```python
from build123d import *

# Parameters (mm, degrees)
ESQUISSE1_W             = 20
ESQUISSE1_H             = 3
BOSS_EXTRU_1_DEPTH      = 3
ESQUISSE2_W             = 172
ESQUISSE2_H             = 1
ENL_V_MAT_EXTRU_1_DEPTH = 1.5
ESQUISSE4_W             = 3
ESQUISSE4_H             = 20
ENL_V_MAT_EXTRU_2_DEPTH = 207.455986147
ESQUISSE5_W             = 70
ESQUISSE5_H             = 100
BOSS_EXTRU_2_DEPTH      = 25
ESQUISSE6_W             = 62
ESQUISSE6_H             = 22.5
ENL_V_MAT_EXTRU_3_DEPTH = 95
ESQUISSE10_W            = 30
ESQUISSE10_H            = 50
BOSS_EXTRU_3_DEPTH      = 20
ESQUISSE11_W            = 25
ESQUISSE11_H            = 17.5
ENL_V_MAT_EXTRU_5_DEPTH = 47
ESQUISSE12_W            = 8
ESQUISSE12_H            = 22.5
BOSS_EXTRU_5_DEPTH      = 15
ESQUISSE15_W            = 7.5
ESQUISSE15_H            = 20
ENL_V_MAT_EXTRU_7_DEPTH = 15
ENL_V_MAT_EXTRU_8_REACH = 210.324
ESQUISSE17_W            = 9
ESQUISSE17_H            = 15
ENL_V_MAT_EXTRU_9_DEPTH = 10


with BuildPart() as part:
    # Esquisse1 → Boss.-Extru.1 (new body)
    with BuildSketch(Plane.XY):
        with BuildLine():
            Line((-109.499197329, 0), (62.500802671, 0))
            Line((62.500802671, 0), (62.500802671, -175))
            Line((62.500802671, -175), (56.500802671, -175))
            ThreePointArc((56.500802671, -175), (-23.499197329, -130.484780132), (-103.499197329, -175))
            Line((-103.499197329, -175), (-109.499197329, -175))
            Line((-109.499197329, -175), (-109.499197329, 0))
        make_face()
        with Locations((-83.499197329, -123.5)):
            Rectangle(ESQUISSE1_W, ESQUISSE1_H, mode=Mode.SUBTRACT)
        with Locations((-23.499197329, -123.5)):
            Rectangle(ESQUISSE1_W, ESQUISSE1_H, mode=Mode.SUBTRACT)
        with Locations((36.500802671, -123.5)):
            Rectangle(ESQUISSE1_W, ESQUISSE1_H, mode=Mode.SUBTRACT)
    extrude(amount=BOSS_EXTRU_1_DEPTH)

    # Esquisse2 → Enlèv. mat.-Extru.1 (cut)
    with BuildSketch(Plane.XY.offset(3)):
        with Locations((-23.499197329, -1)):
            Rectangle(ESQUISSE2_W, ESQUISSE2_H)
    extrude(amount=-ENL_V_MAT_EXTRU_1_DEPTH, mode=Mode.SUBTRACT)

    # Esquisse4 → Enlèv. mat.-Extru.2 (cut, through all)
    with BuildSketch(Plane.XY.offset(3)):
        with Locations((-107.999197329, -78.25)):
            Rectangle(ESQUISSE4_W, ESQUISSE4_H)
        with Locations((61.000802671, -78.25)):
            Rectangle(ESQUISSE4_W, ESQUISSE4_H)
    extrude(amount=-ENL_V_MAT_EXTRU_2_DEPTH, mode=Mode.SUBTRACT)

    # Esquisse5 → Boss.-Extru.2 (add)
    with BuildSketch(Plane.XY.offset(3)):
        with Locations((-22.499197329, -66.5)):
            Rectangle(ESQUISSE5_W, ESQUISSE5_H)
    extrude(amount=BOSS_EXTRU_2_DEPTH)

    # Esquisse6 → Enlèv. mat.-Extru.3 (cut)
    with BuildSketch(Plane(origin=(0, -16.5, 0), x_dir=(1, 0, 0), z_dir=(0, 1, 0))):
        with Locations((-22.499197329, -14.25)):
            Rectangle(ESQUISSE6_W, ESQUISSE6_H)
    extrude(amount=-ENL_V_MAT_EXTRU_3_DEPTH, mode=Mode.SUBTRACT)

    # Esquisse10 → Boss.-Extru.3 (add)
    with BuildSketch(Plane.XY.offset(3)):
        with Locations((-72.499197329, -91.5)):
            Rectangle(ESQUISSE10_W, ESQUISSE10_H)
    extrude(amount=BOSS_EXTRU_3_DEPTH)

    # Esquisse11 → Enlèv. mat.-Extru.5 (cut)
    with BuildSketch(Plane(origin=(0, -66.5, 0), x_dir=(1, 0, 0), z_dir=(0, 1, 0))):
        with Locations((-72.499197329, -11.75)):
            Rectangle(ESQUISSE11_W, ESQUISSE11_H)
    extrude(amount=-ENL_V_MAT_EXTRU_5_DEPTH, mode=Mode.SUBTRACT)

    # Esquisse12 → Boss.-Extru.5 (add)
    with BuildSketch(Plane(origin=(12.500802671, 0, 0), x_dir=(0, 0, -1), z_dir=(1, 0, 0))):
        with Locations((-7, -100.25)):
            Rectangle(ESQUISSE12_W, ESQUISSE12_H)
    extrude(amount=BOSS_EXTRU_5_DEPTH)

    # Esquisse15 → Enlèv. mat.-Extru.7 (cut)
    with BuildSketch(Plane.ZY.offset(-8.500802671)):
        with Locations((6.75, -100.25)):
            Rectangle(ESQUISSE15_W, ESQUISSE15_H)
    extrude(amount=-ENL_V_MAT_EXTRU_7_DEPTH, mode=Mode.SUBTRACT)

    # Esquisse17 → Enlèv. mat.-Extru.8 (cut, up to next)
    with BuildSketch(Plane(origin=(0, 0, 0), x_dir=(-1, 0, 0), z_dir=(0, 0, -1)), mode=Mode.PRIVATE) as enl_v_mat_extru_8_sk1:
        with Locations((-19.000802671, -99.5)):
            Rectangle(ESQUISSE17_W, ESQUISSE17_H)
    enl_v_mat_extru_8_tool1 = extrude(enl_v_mat_extru_8_sk1.sketch, amount=-ENL_V_MAT_EXTRU_8_REACH, mode=Mode.PRIVATE) & part.part
    add(enl_v_mat_extru_8_tool1.solids().sort_by_distance((19.000803, -99.5, 0))[0], mode=Mode.SUBTRACT)

    # Esquisse18 → Enlèv. mat.-Extru.9 (cut)
    with BuildSketch(Plane.XY.offset(3)):
        with BuildLine():
            ThreePointArc((-8.555469882, -131.678386461), (-22.519051553, -117.45703568), (-36.740402335, -131.420617351))
            Line((-36.740402335, -131.420617351), (-8.555469882, -131.678386461))
        make_face()
    extrude(amount=-ENL_V_MAT_EXTRU_9_DEPTH, mode=Mode.SUBTRACT)


solid = part.part
```
Geometry check sheet. Reference: the model listing, model coordinates, mm. A direction names the side the tool comes from. Round coordinates to 2 decimals unless told otherwise and drop trailing zeros. Order: outer loops, then holes, each group sorted by start corner. A loop starts at its lowest first (then second) coordinate and runs counter-clockwise, first axis right, second up. Notation, with made-up numbers: (-35.5, 23.25) - (-2.5, 23.25) arc R24 cw to (-2.5, 58.25) - close; hole circle Ø5 at (51, -17). An arc over 180 degrees is marked (long way). Use a Markdown table: item, result. Add a question column.
1) Thickness scan on line 1 along Z through (x, y) = (-46, -59); line 2 along X through (y, z) = (-111, 6); line 3 along Z through (x, y) = (-61, -97.5). Record the ranges inside material, lowest first.
2) Set-up check for faces 1 (the flat face through (-73, -90, 20.5)), 2 (the cylindrical face through (29.15, -146.583, 1.479)), 3 (the flat face through (-28, -16.5, 26)), 4 (the flat face through (20, -89, 7)), 5 (the flat face through (-87.499, -92, 13)): record each of +Z, -Z, +X, -X, +Y, -Y from which the full face is reachable in a straight line by a thin tool's end or side.
3) Section check B-B (x = 44.5). Record the cut outline in (y, z), then the cut area to 3 significant figures.
4) Mould release check, pull along Y, two halves, no side actions. Record for faces 6 (the flat face through (-23, -111.5, 14)), 7 (the cylindrical face through (-74.477, -145.481, 1.479)), 8 (the flat face through (-23, -63, 25.5)), 9 (the flat face through (16, -110.25, 7)): released by +Y, released by -Y, zero draft, split by the parting line, or undercut.
5) Section check C-C (y = -157). Record the cut outline in (x, z).
6) Section check D-D (x = 19). Record the cut outline in (y, z), then the cut area to 3 significant figures.
7) Gauge pin test, flat ends, axial feed: P1, Ø7.5, axis at y = -87.5, z = 12, coming from the -X side; P2, Ø8, axis at y = -67.5, z = 18.5, coming from the +X side; P3, Ø6, axis at x = -9.5, z = 15, coming from the +Y side. Record the tip position at first contact, or that the pin passes through.
8) Section check A-A (y = -72). Record the cut outline in (x, z), then the cut area to 3 significant figures.
Established:
| question | item | result |
|---|---|---|
| 1 | line 1 | 0 to 3, 25.5 to 28 |
| 1 | line 2 | -87.5 to -85, -60 to -53.5, 8.5 to 27.5 |
| 1 | line 3 | 0 to 3, 20.5 to 23 |
| 2 | face 1 | +Y |
| 2 | face 2 | +Z, -Z, -Y |
| 2 | face 3 | +Z, +X, -X, +Y |
| 2 | face 4 | +Z, +X, +Y |
| 2 | face 5 | +Z, -X, +Y, -Y |
| 3 | outline | (-159.52, 0) - (-125, 0) - (-125, 3) - (-159.52, 3) - close; (-122, 0) - (0, 0) - (0, 3) - (-0.5, 3) - (-0.5, 1.5) - (-1.5, 1.5) - (-1.5, 3) - (-122, 3) - close |
| 3 | area | 468 mm2 |
| 4 | face 6 | released by +Y |
| 4 | face 7 | released by -Y |
| 4 | face 8 | zero draft |
| 4 | face 9 | undercut |
| 5 | outline | (-109.5, 0) - (-88.99, 0) - (-88.99, 3) - (-109.5, 3) - close; (41.99, 0) - (62.5, 0) - (62.5, 3) - (41.99, 3) - close |
| 6 | outline | (-140.62, 0) - (-107, 0) - (-107, 3) - (-110.25, 3) - (-110.25, 10.5) - (-90.25, 10.5) - (-90.25, 3) - (-92, 3) - (-92, 0) - (0, 0) - (0, 3) - (-0.5, 3) - (-0.5, 1.5) - (-1.5, 1.5) - (-1.5, 3) - (-89, 3) - (-89, 11) - (-111.5, 11) - (-111.5, 3) - (-140.62, 3) - close |
| 6 | area | 405 mm2 |
| 7 | P1 | x = -87.5 |
| 7 | P2 | x = 12.5 |
| 7 | P3 | y = -111.5 |
| 8 | outline | (-106.5, 0) - (59.5, 0) - (59.5, 3) - (12.5, 3) - (12.5, 28) - (-57.5, 28) - (-57.5, 23) - (-87.5, 23) - (-87.5, 3) - (-106.5, 3) - close; hole (-85, 3) - (-60, 3) - (-60, 20.5) - (-85, 20.5) - close; hole (-53.5, 3) - (8.5, 3) - (8.5, 25.5) - (-53.5, 25.5) - close |
| 8 | area | 1,020 mm2 |
